from build123d import *

# Parameters (mm, degrees)
SKETCH1_R                 = 4
SKETCH1_R_2               = 2.527736539
BOSS_EXTRUDE1_DEPTH       = 6.35
F_5_0MM_DOWEL_SLOT1_DEPTH = 6.35
SKETCH4_R                 = 8
CUT_EXTRUDE1_DEPTH        = 3.175


# Read off the part's stored shape, not the designer's step: Ø5.0mm Dowel Slot1
with BuildPart() as part:
    # Sketch1 → Boss-Extrude1 (new body)
    with BuildSketch(Plane.XY):
        with BuildLine():
            Line((8, -57.58012907), (-20.66, -57.58012907))
            ThreePointArc((-20.66, -57.58012907), (-22.435973202, -57.254090899), (-23.980332383, -56.318496743))
            Line((-23.980332383, -56.318496743), (-58.320332383, -25.818496743))
            ThreePointArc((-58.320332383, -25.818496743), (-59.560792799, -24.12931648), (-60, -22.08012907))
            Line((-60, -22.08012907), (-60, -17.08012907))
            ThreePointArc((-60, -17.08012907), (-59.560792799, -15.03094166), (-58.320332383, -13.341761396))
            Line((-58.320332383, -13.341761396), (-23.980332383, 17.158238604))
            ThreePointArc((-23.980332383, 17.158238604), (-22.435973202, 18.09383276), (-20.66, 18.41987093))
            Line((-20.66, 18.41987093), (8, 18.41987093))
            ThreePointArc((8, 18.41987093), (9.414213562, 17.834084493), (10, 16.41987093))
            Line((10, 16.41987093), (10, -6.725270109))
            ThreePointArc((10, -6.725270109), (10.152279768, -7.490730718), (10.585929943, -8.139627163))
            Line((10.585929943, -8.139627163), (19.414070057, -16.965975896))
            ThreePointArc((19.414070057, -16.965975896), (19.847720232, -17.614872341), (20, -18.38033295))
            Line((20, -18.38033295), (20, -20.77992519))
            ThreePointArc((20, -20.77992519), (19.847720232, -21.545385798), (19.414070057, -22.194282243))
            Line((19.414070057, -22.194282243), (10.585929943, -31.020630977))
            ThreePointArc((10.585929943, -31.020630977), (10.152279768, -31.669527422), (10, -32.43498803))
            Line((10, -32.43498803), (10, -55.58012907))
            ThreePointArc((10, -55.58012907), (9.414213562, -56.994342632), (8, -57.58012907))
        make_face()
        with Locations((-20.66, -19.58012907)):
            Circle(SKETCH1_R, mode=Mode.SUBTRACT)
        with Locations((-54.318282784, -19.58012907)):
            Circle(SKETCH1_R_2, mode=Mode.SUBTRACT)
        with Locations((-20.66, 14.050414337)):
            Circle(SKETCH1_R_2, mode=Mode.SUBTRACT)
        with Locations((12.998282784, -19.58012907)):
            Circle(SKETCH1_R_2, mode=Mode.SUBTRACT)
        with Locations((-20.66, -53.238409212)):
            Circle(SKETCH1_R_2, mode=Mode.SUBTRACT)
    extrude(amount=BOSS_EXTRUDE1_DEPTH)

    # Ø5.0mm Dowel Slot1 outline → Ø5.0mm Dowel Slot1 (cut)
    with BuildSketch(Plane.XY):
        with BuildLine():
            ThreePointArc((3.85, -22.567426083), (5.629646398, -21.823233219), (6.349772676, -20.033713042))
            ThreePointArc((6.349772676, -20.033713042), (5.629646398, -18.244192864), (3.85, -17.5))
            Line((3.85, -17.5), (-3.85, -17.5))
            ThreePointArc((-3.85, -17.5), (-5.629646398, -18.244192864), (-6.349772676, -20.033713042))
            ThreePointArc((-6.349772676, -20.033713042), (-5.629646398, -21.823233219), (-3.85, -22.567426083))
            Line((-3.85, -22.567426083), (3.85, -22.567426083))
        make_face()
        with BuildLine():
            Line((-3.85, -2.5), (3.85, -2.5))
            ThreePointArc((3.85, -2.5), (6.35, 0), (3.85, 2.5))
            Line((3.85, 2.5), (-3.85, 2.5))
            ThreePointArc((-3.85, 2.5), (-6.35, 0), (-3.85, -2.5))
        make_face()
        with BuildLine():
            Line((-3.85, -42.5), (3.85, -42.5))
            ThreePointArc((3.85, -42.5), (6.35, -40), (3.85, -37.5))
            Line((3.85, -37.5), (-3.85, -37.5))
            ThreePointArc((-3.85, -37.5), (-6.35, -40), (-3.85, -42.5))
        make_face()
    extrude(amount=F_5_0MM_DOWEL_SLOT1_DEPTH, mode=Mode.SUBTRACT)

    # Sketch4 → Cut-Extrude1 (cut)
    with BuildSketch(Plane(origin=(0, 0, 0), x_dir=(-1, 0, 0), z_dir=(0, 0, -1))):
        with Locations((20.66, -19.58012907)):
            Circle(SKETCH4_R)
    extrude(amount=-CUT_EXTRUDE1_DEPTH, mode=Mode.SUBTRACT)


solid = part.part
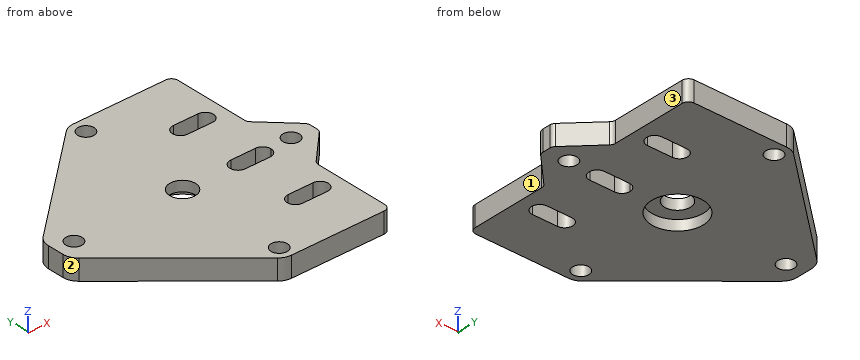
Source: CAD feature listing. Evaluate the final solid. Frame: model axes, mm. Face numbers are marked on the shaded views. A direction names the side the tool comes from. Round coordinates to 2 decimals unless told otherwise and drop trailing zeros. Loops run counter-clockwise (first coordinate to the right, second up) from the corner with the lowest first, then second, coordinate; pieces in that order, holes last. Notation, with made-up numbers: (20.25, 35.5) -> (52.25, 35.5) arc R10 ccw to (52.25, 54.5) -> close; hole circle Ø1 at (50.25, -38). An arc over 180 degrees is marked (long way). Answer as a JSON object with one key per item and string values. Group by question number.
Q1. Section query C-C (x = -44). Output: boundary loops of the cut face in (y, z).
Q2. Section query D-D (y = 0). Output: boundary loops of the cut face in (x, z), plus the area to 3 significant figures.
Q3. Contact query for flat-ended pins moving along their axis: P1, Ø1.5, axis at y = -31, z = 5, coming from the +X side; P2, Ø1, axis at y = -32.5, z = 4.5, coming from the -X side; P3, Ø3, axis at y = -33.5, z = 5, coming from the +X side. Output: stop coordinate, or through.
Q4. Ray query, line 1 (Y direction, x = -20.66, z = 5.15); line 2 (Y direction, x = -1.5, z = 5.25); line 3 (X direction, y = -18.5, z = 5.25). Return the intervals inside material, ascending. Write a range as from..to.
Q5. Section query A-A (y = -39). Output: boundary loops of the cut face in (x, z), plus the area to 3 significant figures.
Q6. Access query for the marked faces 1, 2 and 3. Directions: +Z, -Z, +X, -X, +Y, -Y. A direction counts if a zero-diameter tool reaches every point of the face in a straight line with its end or side. Return the directions, or none.
Q7. Section query B-B (z = 4.75). State how many separate pieces and enclosed holes the cut face has, plus the area to 3 significant figures.
Completed:
{
 "1": {"outline": "(-38.54, 0) -> (-0.62, 0) -> (-0.62, 6.35) -> (-38.54, 6.35) -> close"},
 "2": {"outline": "(-43.3, 0) -> (-6.35, 0) -> (-6.35, 6.35) -> (-43.3, 6.35) -> close; (6.35, 0) -> (10, 0) -> (10, 6.35) -> (6.35, 6.35) -> close", "area": "258 mm²"},
 "3": {"P1": "x = 11.36", "P2": "x = -51.36", "P3": "x = 10.05"},
 "4": {"line 1": "-57.58..-55.77, -50.71..-23.58, -15.58..11.52, 16.58..18.42", "line 2": "-57.58..-42.5, -37.5..-22.57, -17.5..-2.5, 2.5..18.42", "line 3": "-60..-56.6, -52.03..-24.51, -16.81..-5.85, 5.85..10.71, 15.28..20"},
 "5": {"outline": "(-43.48, 0) -> (-6.14, 0) -> (-6.14, 6.35) -> (-43.48, 6.35) -> close; (6.14, 0) -> (10, 0) -> (10, 6.35) -> (6.14, 6.35) -> close", "area": "262 mm²"},
 "6": {"face 1": "+Z, -Z, +X, -Y", "face 2": "+Z, -Z, -X, -Y", "face 3": "+Z, -Z, +X, +Y"},
 "7": {"separate pieces": "1", "enclosed holes": "8", "area": "3,910 mm²"}
}
